```python
from build123d import *

# Parameters (mm, degrees)
SKETCH1_R           = 1.35
SKETCH1_R_2         = 12.095
SKETCH1_R_3         = 1.143
SKETCH1_W           = 11
SKETCH1_H           = 69
BOSS_EXTRUDE2_DEPTH = 3.175
FILLET1_R           = 2


with BuildPart() as part:
    # Sketch1 → Boss-Extrude2 (new body)
    with BuildSketch(Plane(origin=(0, 0, 0), x_dir=(1, 0, 0), z_dir=(0, 1, 0))):
        with BuildLine():
            ThreePointArc((32.995567884, -67.352004425), (0, 75), (-32.995567884, -67.352004425))
            ThreePointArc((-32.995567884, -67.352004425), (0, -48.302004425), (32.995567884, -67.352004425))
        make_face()
        with Locations((-42.910067426, 11.1)):
            Circle(SKETCH1_R, mode=Mode.SUBTRACT)
        with Locations((-42.910067426, -11.1)):
            Circle(SKETCH1_R, mode=Mode.SUBTRACT)
        with Locations((-11.160067426, -11.1)):
            Circle(SKETCH1_R, mode=Mode.SUBTRACT)
        with Locations((-11.160067426, 11.1)):
            Circle(SKETCH1_R, mode=Mode.SUBTRACT)
        with Locations((11.160067426, 11.1)):
            Circle(SKETCH1_R, mode=Mode.SUBTRACT)
        with Locations((11.160067426, -11.1)):
            Circle(SKETCH1_R, mode=Mode.SUBTRACT)
        with Locations((42.910067426, -11.1)):
            Circle(SKETCH1_R, mode=Mode.SUBTRACT)
        with Locations((42.910067426, 11.1)):
            Circle(SKETCH1_R, mode=Mode.SUBTRACT)
        with Locations((26.905821676, -20.904643604)):
            Circle(SKETCH1_R_2, mode=Mode.SUBTRACT)
        with Locations((19, 49)):
            Circle(SKETCH1_R_2, mode=Mode.SUBTRACT)
        with Locations((0, 29.793589551)):
            Circle(SKETCH1_R_2, mode=Mode.SUBTRACT)
        with Locations((0, -25.409190322)):
            Circle(SKETCH1_R_2, mode=Mode.SUBTRACT)
        with Locations((29.939937248, 24.651901309)):
            Circle(SKETCH1_R_2, mode=Mode.SUBTRACT)
        with Locations((-26.905821676, -20.904643604)):
            Circle(SKETCH1_R_2, mode=Mode.SUBTRACT)
        with Locations((6.731, 61.422565207)):
            Circle(SKETCH1_R_3, mode=Mode.SUBTRACT)
        with Locations((-6.731, 61.422565207)):
            Circle(SKETCH1_R_3, mode=Mode.SUBTRACT)
        with Locations((-29.939937248, 24.651901309)):
            Circle(SKETCH1_R_2, mode=Mode.SUBTRACT)
        with Locations((-33.21799214, 49)):
            Circle(SKETCH1_R, mode=Mode.SUBTRACT)
        with Locations((-4.78200786, 49)):
            Circle(SKETCH1_R, mode=Mode.SUBTRACT)
        with Locations((4.78200786, 49)):
            Circle(SKETCH1_R, mode=Mode.SUBTRACT)
        with Locations((-42.910067426, 18.234848025)):
            Circle(SKETCH1_R, mode=Mode.SUBTRACT)
        with Locations((42.910067426, 18.234848025)):
            Circle(SKETCH1_R, mode=Mode.SUBTRACT)
        with Locations((-19, 49)):
            Circle(SKETCH1_R_2, mode=Mode.SUBTRACT)
        with Locations((45.13872464, 31.997163897)):
            Circle(SKETCH1_R, mode=Mode.SUBTRACT)
        with Locations((-45.13872464, 31.997163897)):
            Circle(SKETCH1_R, mode=Mode.SUBTRACT)
        with Locations((13.346873881, 34.693819966)):
            Circle(SKETCH1_R, mode=Mode.SUBTRACT)
        with Locations((-6.55476095, -38.026099982)):
            Circle(SKETCH1_R, mode=Mode.SUBTRACT)
        with Locations((-13.346873881, 34.693819966)):
            Circle(SKETCH1_R, mode=Mode.SUBTRACT)
        with Locations((10.597026674, -15.930038136)):
            Circle(SKETCH1_R, mode=Mode.SUBTRACT)
        with Locations((-38.234289702, -39.23697625)):
            Circle(SKETCH1_R, mode=Mode.SUBTRACT)
        with Locations((-43.735655662, -41.075447944)):
            Circle(SKETCH1_R, mode=Mode.SUBTRACT)
        with Locations((-43.735655662, 41.075447944)):
            Circle(SKETCH1_R, mode=Mode.SUBTRACT)
        with Locations((43.735655662, -41.075447944)):
            Circle(SKETCH1_R, mode=Mode.SUBTRACT)
        with Locations((33.21799214, 49)):
            Circle(SKETCH1_R, mode=Mode.SUBTRACT)
        with Locations((43.735655662, 41.075447944)):
            Circle(SKETCH1_R, mode=Mode.SUBTRACT)
        with Locations((-44.385223141, -22.074211772)):
            Circle(SKETCH1_R, mode=Mode.SUBTRACT)
        with Locations((41.601681906, -17.457756634)):
            Circle(SKETCH1_R, mode=Mode.SUBTRACT)
        with Locations((38.234289702, -39.23697625)):
            Circle(SKETCH1_R, mode=Mode.SUBTRACT)
        with Locations((58.910067426, 0.102907352)):
            Rectangle(SKETCH1_W, SKETCH1_H, mode=Mode.SUBTRACT)
        with Locations((-58.910067426, 0.102907352)):
            Rectangle(SKETCH1_W, SKETCH1_H, mode=Mode.SUBTRACT)
    extrude(amount=BOSS_EXTRUDE2_DEPTH)

    # Fillet1
    fillet1_edges = [part.edges().sort_by_distance(p)[0] for p in [
        (-32.995567884, 1.5875, 67.352004425),
        (32.995567884, 1.5875, 67.352004425),
    ]]
    fillet(fillet1_edges, radius=FILLET1_R)


solid = part.part
```
CAD build for the part. Positions are in the model's coordinates, mm. Give positions to 0.01 mm unless a question says otherwise; leave off trailing zeros. Order: outer loops, then holes, each group sorted by start corner. A loop starts at its lowest first (then second) coordinate and runs counter-clockwise, first axis right, second up. Notation, with made-up numbers: M 53.25,-40 L 61.25,-40 A14 cw 61.25,-13 Z; hole C 53,83.5 d1. An arc over 180 degrees is marked long. Put each result on its own line as item: value. Start each with the question number.
(1) Saw through at B-B, the plane z = 1.5. Write the cut outline in (x, y) (3 decimals), then the cut area to 3 significant figures.
(2) Saw through at C-C, the plane z = -27. Write the cut outline in (x, y) (3 decimals), then the cut area to 3 significant figures.
(3) Drill centre lines: line 1 along Z through (x, y) = (19, 2.85) (3 decimals); line 2 along X through (y, z) = (1.15, 29); line 3 along X through (y, z) = (1.4, -56.5). Where is each one in solid material? Low to high.
(4) Flat gauge pins, fed straight in: pin 1 Ø1 at (x, y) = (33, 2) entering from -Z; pin 2 Ø1 at (y, z) = (2.5, -10.5) entering from +X. Where does each tip first touch, or does it go through?
(5) Mould opens along Z. For faces 1 (the flat face through (64.41, 2, 0)), 2 (the cylindrical face through (-0.533, 1.565, 48.306)), 3 (the cylindrical face through (2.79, 1.57, -74.95)), 4 (the flat face through (-1, 3.175, -5)) say: +Z half, -Z half, draft (parallel to the pull), parting line (faces both ways), or undercut.
(6) Saw through at A-A, the plane x = -60.5. Write the cut outline in (y, z) (1 decimal), then the cut area to 3 significant figures.
(7) Saw through at D-D, the plane y = 1.05. Give the number of separate pieces and of enclosed holes in the cut face, then the cut area to 3 significant figures.
Check result:
1. outline: M -74.985,0 L -64.41,0 L -64.41,3.175 L -74.985,3.175 Z; M -53.41,0 L 53.41,0 L 53.41,3.175 L -53.41,3.175 Z; M 64.41,0 L 74.985,0 L 74.985,3.175 L 64.41,3.175 Z
1. area: 406 mm2
2. outline: M -69.971,0 L -64.41,0 L -64.41,3.175 L -69.971,3.175 Z; M -53.41,0 L -41.805,0 L -41.805,3.175 L -53.41,3.175 Z; M -18.075,0 L -11.768,0 L -11.768,3.175 L -18.075,3.175 Z; M 11.768,0 L 18.075,0 L 18.075,3.175 L 11.768,3.175 Z; M 41.805,0 L 53.41,0 L 53.41,3.175 L 41.805,3.175 Z; M 64.41,0 L 69.971,0 L 69.971,3.175 L 64.41,3.175 Z
2. area: 149 mm2
3. line 1: z = -72.553 to -61.095, -36.905 to -29.81, -19.494 to 11.751, 30.058 to 53.378
3. line 2: x = -69.17 to -64.41, -53.41 to -35.89, -17.92 to -11.55, 11.55 to 17.92, 35.89 to 53.41, 64.41 to 69.17
3. line 3: x = -49.32 to -28.49, -9.51 to 9.51, 28.49 to 49.32
4. pin 1: stops at z = -67.59
4. pin 2: stops at x = 74.33
5. face 1: undercut
5. face 2: +Z half
5. face 3: parting line
5. face 4: draft
6. outline: M 0,-44.3 L 3.2,-44.3 L 3.2,-34.6 L 0,-34.6 Z; M 0,34.4 L 3.2,34.4 L 3.2,44.3 L 0,44.3 Z
6. area: 62.4 mm2
7. separate pieces: 1
7. enclosed holes: 40
7. area: 11,100 mm2
